Could you check a few things on this drawing? It's one solid part, dimensions in mm from its lowest x, y, z. A direction names the side the tool comes from. Coordinates: 2 decimals unless noted, no trailing zeros. Write each loop counter-clockwise with the first axis right and the second up, starting at its lowest first coordinate (ties: lowest second). Pieces come first, ordered by that corner, then holes. Notation, with made-up numbers: M -21,64.25 L -10,64.25 A14 ccw -10,83.25 Z; hole C -22.5,18 d10. An arc over 180 degrees is marked long. Use a Markdown table: item, result.
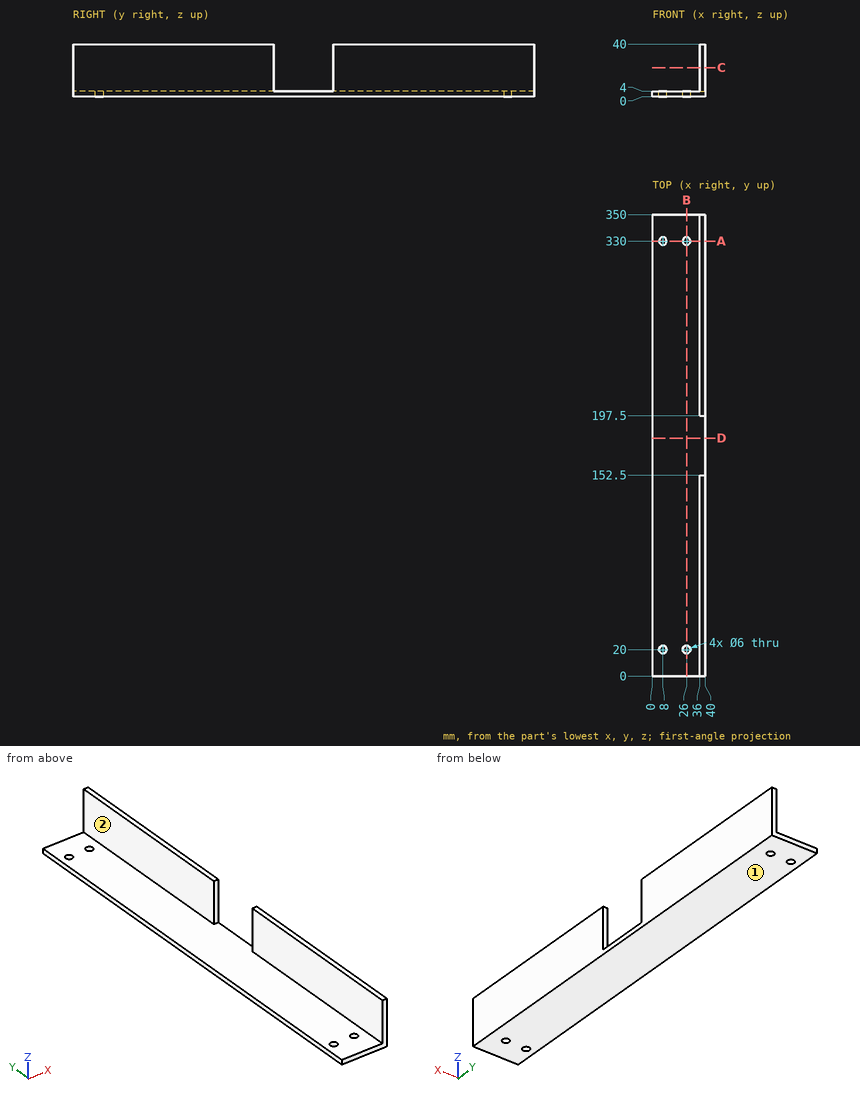
1. Suppose I cut it at C-C on z = 22. Write out the boundary of the cut face in (x, y), and give its area (3 significant figures).
Answers follow:
| item | result |
|---|---|
| outline | M 36,0 L 40,0 L 40,152.5 L 36,152.5 Z; M 36,197.5 L 40,197.5 L 40,350 L 36,350 Z |
| area | 1,220 mm2 |
2. I need wall thicknesses on probe 1 along X at (y, z) = (20, 2.7); probe 2 along Z at (x, y) = (14.5, 238.5); probe 3 along X at (y, z) = (108, 31). Which ranges of each line are inside material? Lowest first, please.
Answers follow:
| item | result |
|---|---|
| probe 1 | x = 0 to 5, 11 to 23, 29 to 40 |
| probe 2 | z = 0 to 4 |
| probe 3 | x = 36 to 40 |
3. Suppose I cut it at A-A on y = 330. Write out the boundary of the cut face in (x, z), and give its area (3 significant figures).
Answers follow:
| item | result |
|---|---|
| outline | M 0,0 L 5,0 L 5,4 L 0,4 Z; M 11,0 L 23,0 L 23,4 L 11,4 Z; M 29,0 L 40,0 L 40,40 L 36,40 L 36,4 L 29,4 Z |
| area | 256 mm2 |
4. Suppose I cut it at B-B on x = 26. Write out the boundary of the cut face in (y, z), and give its area (3 significant figures).
Answers follow:
| item | result |
|---|---|
| outline | M 0,0 L 17,0 L 17,4 L 0,4 Z; M 23,0 L 327,0 L 327,4 L 23,4 Z; M 333,0 L 350,0 L 350,4 L 333,4 Z |
| area | 1,350 mm2 |
5. Suppose I cut it at D-D on y = 180.5. Write out the boundary of the cut face in (x, z).
Answers follow:
| item | result |
|---|---|
| outline | M 0,0 L 40,0 L 40,4 L 0,4 Z |
6. Which directions (+Z, -Z, +X, -X, +Y, -Y) give clear straight access to the entire face, cutting with the end or side of a thin tool? Please do the marked faces 1 and 2.
Answers follow:
| item | result |
|---|---|
| face 1 | -Z, +X, -X, +Y, -Y |
| face 2 | +Z, -X, +Y, -Y |
